Autodesk Inventor part; units mm, degrees
ref_plane "YZ Plane" through (0, 0, 0) normal (1, 0, 0) x (0, 1, 0)
ref_plane "XZ Plane" through (0, 0, 0) normal (0, 1, 0) x (-1, 0, 0)
ref_plane "XY Plane" through (0, 0, 0) normal (0, 0, 1) x (1, 0, 0)
sketch "Sketch1" plane through (0, 0, 0) normal (0, 1, 0) x (-1, 0, 0)
  circle A0 centre (0, 0) radius 35
  dimension "d0" = 70
extrude "Extrusion1" add sketch "Sketch1" along normal blind 2
sketch "Sketch2" plane through (0, 2, 0) normal (0, 1, 0) x (1, 0, 0)
  circle A0 centre (0, 0) radius 7.5
  dimension "d3" = 15
extrude "Extrusion2" add sketch "Sketch2" along normal blind 5
sketch "Sketch3" plane through (0, 0, 0) normal (0, -1, 0) x (1, 0, 0)
  line L0 (22.7941, 0) -> (-22.7941, 0) construction
  line L1 (0, 29.7059) -> (0, -29.7059) construction
  point P0 (0, 0)
  point P1 (20, 20)
  point P2 (20, -20)
  point P3 (-20, -20)
  point P4 (-20, 20)
  point P5 (0, 0)
  dimension "d6" = 40
  dimension "d7" = 40
  dimension "d8" = 20
  dimension "d9" = 20
hole "Hole1" at (20, 0, 20) at (20, 0, -20) at (-20, 0, -20) at (-20, 0, 20) direction (0, 1, 0) diameter 5.5 end through all
properties part number "FlanschSchablone"
For this review, take the finished solid that the model builds, in its own axes (mm). Round coordinates to 2 decimals unless told otherwise and drop trailing zeros. Loops run counter-clockwise (first coordinate to the right, second up) from the corner with the lowest first, then second, coordinate; pieces in that order, holes last. Notation, with made-up numbers: (-5.5, 71) - (33.5, 71) arc R28 cw to (33.5, 91) - close; hole circle Ø7 at (-29, 14). An arc over 180 degrees is marked (long way). One line per question, with ' | ' between items.
Q1. Take a section at D-D (z = 4.5). Give the boundary of the cut face in (x, y), and give its area (3 significant figures).
Taken from the geometry:
outline: (-34.71, 0) - (34.71, 0) - (34.71, 2) - (6, 2) - (6, 7) - (-6, 7) - (-6, 2) - (-34.71, 2) - close | area: 199 mm²
Q2. For line 1 along Z through (x, y) = (20, 0.55); line 2 along Z through (x, y) = (-18, 1.5), list the stretches that pass through material, from the lowest coordinate up. Write a range as [from, to].
Taken from the geometry:
line 1: z = [-28.72, -22.75], [-17.25, 17.25], [22.75, 28.72] | line 2: z = [-30.02, -21.89], [-18.11, 18.11], [21.89, 30.02]
Q3. Take a section at C-C (x = 0). Give the boundary of the cut face in (y, z), and give its area (3 significant figures).
Taken from the geometry:
outline: (0, -35) - (2, -35) - (2, -7.5) - (7, -7.5) - (7, 7.5) - (2, 7.5) - (2, 35) - (0, 35) - close | area: 215 mm²
Q4. Take a section at A-A (z = 18.5). Give the boundary of the cut face in (x, y), and give its area (3 significant figures).
Taken from the geometry:
outline: (-29.71, 0) - (-22.3, 0) - (-22.3, 2) - (-29.71, 2) - close; (-17.7, 0) - (17.7, 0) - (17.7, 2) - (-17.7, 2) - close; (22.3, 0) - (29.71, 0) - (29.71, 2) - (22.3, 2) - close | area: 100 mm²
Q5. Take a section at B-B (x = 20). Give the boundary of the cut face in (y, z), and give its area (3 significant figures).
Taken from the geometry:
outline: (0, -28.72) - (2, -28.72) - (2, -22.75) - (0, -22.75) - close; (0, -17.25) - (2, -17.25) - (2, 17.25) - (0, 17.25) - close; (0, 22.75) - (2, 22.75) - (2, 28.72) - (0, 28.72) - close | area: 92.9 mm²
Q6. For pin 1 (1 mm diameter, centred on x = 6, y = 2, fed in from +Z); pin 2 (3 mm diameter, centred on y = 3, z = 9, fed in from -X); pin 3 (1.5 mm diameter, centred on x = 3, z = -20.5, fed in from +Y), all flat-tipped, find the tip position at first contact; note any pin that passes through.
Taken from the geometry:
pin 1: stops at z = 34.57 | pin 2: stops at x = -34.1 | pin 3: stops at y = 2
Q7. The part is to be moulded in two halves that separate along X. For faces 1 (the flat face through (0, 7, 0)), 2 (the cylindrical face through (-7.493, 4.465, 0.33)), 3 (the cylindrical face through (-20.121, 1.014, 22.747)), say which applies: released by +X, released by -X, zero draft, split by the parting line, or undercut.
Taken from the geometry:
face 1: zero draft | face 2: split by the parting line | face 3: undercut
